For this review, take the finished solid that the model builds, in its own axes (mm). Face numbers are marked on the shaded views. Coordinates: 2 decimals unless noted, no trailing zeros. Write each loop counter-clockwise with the first axis right and the second up, starting at its lowest first coordinate (ties: lowest second). Pieces come first, ordered by that corner, then holes. Notation, with made-up numbers: (52.5, -35.5) -> (97.5, -35.5) arc R32 ccw to (97.5, -9.5) -> close; hole circle Ø7 at (82.25, -8). An arc over 180 degrees is marked (long way). Put each result on its own line as item: value. Start each with the question number.
Item 1: Consider section B-B on z = 13.95. Give the boundary of the cut face in (x, y), and give its area (3 significant figures).
Item 2: The part is to be moulded in two halves that separate along X. For the marked faces 1, 2, 3 and 4, say which applies: +X half, -X half, draft (parallel to the pull), parting line (faces both ways), or undercut.
Item 3: Consider section A-A on x = 7.85. Give the boundary of the cut face in (y, z), and give its area (3 significant figures).
Item 4: Consider section C-C on y = 0.65. Give the boundary of the cut face in (x, z).
Item 5: Consider section D-D on x = -4.05. Give the boundary of the cut face in (y, z).
Item 6: Insertion check: P1, Ø4.5, axis at x = -4.1, z = -18.05, coming from the -Y side. The pin has a flat end and moves straight along its axis. Give the tip position at first contact, or say it passes through.
Item 7: To check wall thickness, follow L1, parallel to Z at x = -4.1, y = 3.25; L2, parallel to Z at x = -16, y = 2.95; L3, parallel to Z at x = -2.5, y = 4.9. State the ranges of each line that lie inside material, in increasing order.
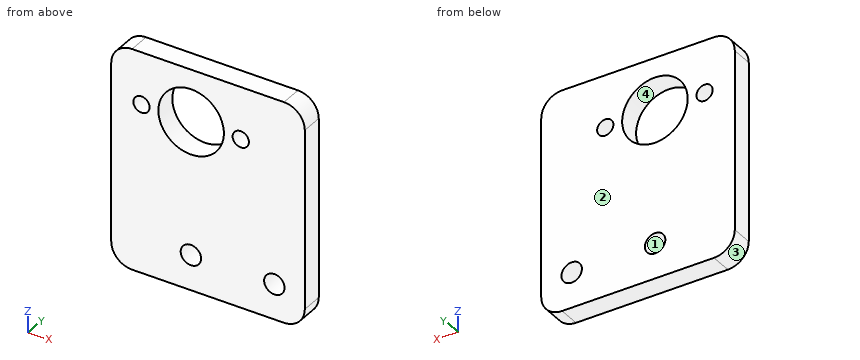
Autodesk Inventor part; units mm, degrees
ref_plane "YZ Plane" through (0, 0, 0) normal (1, 0, 0) x (0, 1, 0)
ref_plane "XZ Plane" through (0, 0, 0) normal (0, 1, 0) x (-1, 0, 0)
ref_plane "XY Plane" through (0, 0, 0) normal (0, 0, 1) x (1, 0, 0)
sketch "Boceto1" plane through (0, 0, 0) normal (0, 1, 0) x (-1, 0, 0)
  line L0 (-23.2, -26.5) -> (23.2, -26.5)
  line L1 (23.2, -26.5) -> (23.2, 26.5)
  line L2 (23.2, 26.5) -> (-23.2, 26.5)
  line L3 (-23.2, 26.5) -> (-23.2, -26.5)
  line L4 (-23.2, -26.5) -> (23.2, 26.5) construction
  line L5 (23.2, -26.5) -> (-23.2, 26.5) construction
  line L6 (23.2, 26.5) -> (23.2, 21.8)
  line L7 (23.2, 21.8) -> (-23.2, 21.8)
  line L8 (23.2, 21.8) -> (11.9, 21.8)
  line L9 (11.9, 21.8) -> (11.9, 0)
  circle A0 centre (4.05, 13.95) radius 7.85
  line L10 (11.9, 13.95) -> (14, 13.95)
  line L11 (14, 13.95) -> (15.95, 13.95)
  circle A1 centre (15.95, 13.95) radius 1.95
  line L12 (-3.8, 13.95) -> (-5.9, 13.95)
  line L13 (-5.9, 13.95) -> (-7.85, 13.95)
  circle A2 centre (-7.85, 13.95) radius 1.95
  line L14 (23.2, -26.5) -> (23.2, -20.5)
  line L15 (23.2, -20.5) -> (-23.2, -20.5)
  line L16 (23.2, -20.5) -> (6.55, -20.5)
  line L17 (6.55, -20.5) -> (1.65, -20.5)
  line L18 (4.1, -20.5) -> (4.1, -18.05)
  circle A3 centre (4.1, -18.05) radius 2.45
  line L19 (1.65, -18.05) -> (-13.45, -18.05)
  line L20 (-13.45, -18.05) -> (-15.9, -18.05)
  circle A4 centre (-15.9, -18.05) radius 2.45
  point P0 (0, 0)
  point P1 (4.05, 21.8)
  dimension "d0" = 46.4
  dimension "d1" = 53
  dimension "d2" = 4.7
  dimension "d3" = 11.3
  dimension "d4" = 15.7
  dimension "d5" = 2.1
  dimension "d6" = 1.95
  dimension "d7" = 2.1
  dimension "d8" = 1.95
  dimension "d9" = 6
  dimension "d10" = 16.65
  dimension "d11" = 4.9
  dimension "d12" = 2.45
  dimension "d13" = 15.1
  dimension "d14" = 2.45
extrude "Extrusión1" add sketch "Boceto1" along normal blind 5.2 contours L3 L15 L1 L0 | L3 L7 A0 L9 L1 L15 A3 L19 A4 | L3 L2 L1 L7 | A4 L19 A3 L15 | L7 L9 A0
fillet "Empalme1" radius 5 4 edges at (-23.2, 2.6, 26.5) (-23.2, 2.6, -26.5) (23.2, 2.6, -26.5) (23.2, 2.6, 26.5)
properties part number "soporte eje z"
Return value:
1. outline: (-23.2, 0) -> (-17.9, 0) -> (-17.9, 5.2) -> (-23.2, 5.2) -> close; (-14, 0) -> (-11.9, 0) -> (-11.9, 5.2) -> (-14, 5.2) -> close; (3.8, 0) -> (5.9, 0) -> (5.9, 5.2) -> (3.8, 5.2) -> close; (9.8, 0) -> (23.2, 0) -> (23.2, 5.2) -> (9.8, 5.2) -> close
1. area: 119 mm^2
2. face 1: undercut
2. face 2: draft
2. face 3: -X half
2. face 4: undercut
3. outline: (0, -26.5) -> (5.2, -26.5) -> (5.2, 12) -> (0, 12) -> close; (0, 15.9) -> (5.2, 15.9) -> (5.2, 26.5) -> (0, 26.5) -> close
3. area: 255 mm^2
4. outline: (-23.2, -21.5) arc R5 ccw to (-18.2, -26.5) -> (18.2, -26.5) arc R5 ccw to (23.2, -21.5) -> (23.2, 21.5) arc R5 ccw to (18.2, 26.5) -> (-18.2, 26.5) arc R5 ccw to (-23.2, 21.5) -> close; hole circle Ø3.9 at (-15.95, 13.95); hole circle Ø15.7 at (-4.05, 13.95); hole circle Ø4.9 at (-4.1, -18.05); hole circle Ø3.9 at (7.85, 13.95); hole circle Ø4.9 at (15.9, -18.05)
5. outline: (0, -26.5) -> (5.2, -26.5) -> (5.2, -20.5) -> (0, -20.5) -> close; (0, -15.6) -> (5.2, -15.6) -> (5.2, 6.1) -> (0, 6.1) -> close; (0, 21.8) -> (5.2, 21.8) -> (5.2, 26.5) -> (0, 26.5) -> close
6. P1: through
7. L1: -26.5 to -20.5, -15.6 to 6.1, 21.8 to 26.5
7. L2: -26.5 to 12, 15.9 to 26.5
7. L3: -26.5 to -19.91, -16.19 to 6.25, 21.65 to 26.5
